from build123d import *

# Parameters (mm, degrees)
SKETCH_W        = 86
SKETCH_H        = 24
SKETCH_R        = 1.5
PAD_DEPTH       = 6
SKETCH002_R     = 2
POCKET_DEPTH    = 10
SKETCH003_R     = 2
POCKET001_DEPTH = 10


with BuildPart() as part:
    # Sketch → Pad (new body)
    with BuildSketch(Plane.XY):
        with Locations((43, 12)):
            Rectangle(SKETCH_W, SKETCH_H)
        with Locations((13.999996, 11.999945)):
            Circle(SKETCH_R, mode=Mode.SUBTRACT)
        with Locations((71.999985, 11.999591)):
            Circle(SKETCH_R, mode=Mode.SUBTRACT)
    extrude(amount=PAD_DEPTH)

    # Sketch002 (on Face2 of Pad) → Pocket (cut)
    with BuildSketch(Plane.YZ.offset(86)):
        with Locations((3.999421, 2.998608)):
            Circle(SKETCH002_R)
        with Locations((19.998423, 2.997373)):
            Circle(SKETCH002_R)
    extrude(amount=-POCKET_DEPTH, mode=Mode.SUBTRACT)

    # Sketch003 (on Face2 of Pocket) → Pocket001 (cut)
    with BuildSketch(Plane(origin=(0, 0, 0), x_dir=(0, -1, 0), z_dir=(-1, 0, 0))):
        with Locations((-4.000442, 2.999754)):
            Circle(SKETCH003_R)
        with Locations((-20.000246, 2.999371)):
            Circle(SKETCH003_R)
    extrude(amount=-POCKET001_DEPTH, mode=Mode.SUBTRACT)


solid = part.part
Check sheet for the modelled part. Datum: model origin and axes. Units: mm. A direction names the side the tool comes from. Coordinates: 2 decimals unless noted, no trailing zeros. Loops run counter-clockwise (first coordinate to the right, second up) from the corner with the lowest first, then second, coordinate; pieces in that order, holes last. Notation, with made-up numbers: (20, 72.25) -> (39, 72.25) arc R27 ccw to (39, 93.25) -> close; hole circle Ø5 at (-8, 5). An arc over 180 degrees is marked (long way). Write item = value, one per line. Start each with the question number.
1. Section check C-C on y = 3.25. Record the cut outline in (x, z), then the cut area to 3 significant figures.
2. Section check D-D on y = 19.5. Record the cut outline in (x, z).
3. Material ranges on line 1 (X direction, y = 12, z = 1.1); line 2 (Y direction, x = 78.5, z = 4.5); line 3 (X direction, y = 11, z = 0.9), recorded low to high.
4. Depth check by flat-ended pin: P1, Ø1.2, axis at y = 21, z = 3.5, coming from the +X side; P2, Ø3.5, axis at x = 72, y = 12, coming from the +Z side. Enter the tip coordinate at first touch or a pass-through.
5. Section check B-B on z = 3.9. Record the cut outline in (x, y).
6. Section check A-A on x = 79. Record the cut outline in (y, z), then the cut area to 3 significant figures.
7. Tool access check on faces 4 (the flat face through (0, 12, 3)), 5 (the cylindrical face through (81.07, 18.524, 4.349)), 6 (the cylindrical face through (4.9, 5.6, 1.8)). Record the directions out of +Z, -Z, +X, -X, +Y, -Y that give a thin tool (end or side, any length) a straight path to the whole face; none if there is none.
8. Draft check along Z on faces 1 (the cylindrical face through (4.9, 21.6, 1.8)), 2 (the flat face through (42, 12, 0)), 3 (the flat face through (42, 0, 3)). Enter one of: released by +Z, released by -Z, zero draft, split by the parting line, or undercut.
Responses:
q1.outline = (0, 0) -> (86, 0) -> (86, 1.14) -> (76, 1.14) -> (76, 4.85) -> (86, 4.85) -> (86, 6) -> (0, 6) -> (0, 4.85) -> (10, 4.85) -> (10, 1.15) -> (0, 1.15) -> close
q1.area = 442 mm2
q2.outline = (0, 0) -> (86, 0) -> (86, 1.06) -> (76, 1.06) -> (76, 4.93) -> (86, 4.93) -> (86, 6) -> (0, 6) -> (0, 4.94) -> (10, 4.94) -> (10, 1.06) -> (0, 1.06) -> close
q3.line_1 = 0 to 12.5, 15.5 to 70.5, 73.5 to 86
q3.line_2 = 0 to 2.68, 5.32 to 18.68, 21.32 to 24
q3.line_3 = 0 to 12.88, 15.12 to 70.88, 73.12 to 86
q4.P1 = 76
q4.P2 = 6
q5.outline = (0, 0) -> (86, 0) -> (86, 2.21) -> (76, 2.21) -> (76, 5.78) -> (86, 5.78) -> (86, 18.21) -> (76, 18.21) -> (76, 21.78) -> (86, 21.78) -> (86, 24) -> (0, 24) -> (0, 21.79) -> (10, 21.79) -> (10, 18.21) -> (0, 18.21) -> (0, 5.79) -> (10, 5.79) -> (10, 2.21) -> (0, 2.21) -> close; hole circle Ø3 at (14, 12); hole circle Ø3 at (72, 12)
q6.outline = (0, 0) -> (24, 0) -> (24, 6) -> (0, 6) -> close; hole circle Ø4 at (4, 3); hole circle Ø4 at (20, 3)
q6.area = 119 mm2
q7.face_4 = +Z, -Z, -X, +Y, -Y
q7.face_5 = +X
q7.face_6 = -X
q8.face_1 = undercut
q8.face_2 = released by -Z
q8.face_3 = zero draft
